Geometry check sheet. Reference: the model listing, model coordinates, mm. A direction names the side the tool comes from. Round coordinates to 2 decimals unless told otherwise and drop trailing zeros. Write each loop counter-clockwise with the first axis right and the second up, starting at its lowest first coordinate (ties: lowest second). Pieces come first, ordered by that corner, then holes. Notation, with made-up numbers: (62, 35) - (68, 35) arc R16 ccw to (68, 57) - close; hole circle Ø9 at (55.5, 37). An arc over 180 degrees is marked (long way). One line per question, with ' | ' between items. Start each with the question number.
from build123d import *

# Parameters (mm, degrees)
SKETCH_W     = 23
SKETCH_H     = 15
PAD_DEPTH    = 20
SKETCH001_R  = 2.5
PAD001_DEPTH = 1
SKETCH002_W  = 6
SKETCH002_H  = 25
PAD002_DEPTH = 20


with BuildPart() as part:
    # Sketch → Pad (new body)
    with BuildSketch(Plane.XY):
        with Locations((11.5, 0)):
            Rectangle(SKETCH_W, SKETCH_H)
    extrude(amount=PAD_DEPTH)

    # Sketch001 (on Face5 of Pad) → Pad001 (join)
    with BuildSketch(Plane(origin=(0, 0, 7), x_dir=(1, 0, 0), z_dir=(0, 0, -1))):
        with BuildLine():
            ThreePointArc((8, -13), (12.5, -17.5), (17, -13))
            Line((17, 13), (17, -13))
            ThreePointArc((17, 13), (12.5, 17.5), (8, 13))
            Line((8, -13), (8, 13))
        make_face()
        with Locations((12.5, -13)):
            Circle(SKETCH001_R, mode=Mode.SUBTRACT)
        with Locations((12.5, 13)):
            Circle(SKETCH001_R, mode=Mode.SUBTRACT)
    extrude(amount=-PAD001_DEPTH)

    # Sketch002 (on Face3 of Pad001) → Pad002 (join)
    with BuildSketch(Plane(origin=(0, 0, 0), x_dir=(1, 0, 0), z_dir=(0, 0, -1))):
        with Locations((20, 0)):
            Rectangle(SKETCH002_W, SKETCH002_H)
    extrude(amount=-PAD002_DEPTH)


solid = part.part
Q1. Go/stop test with flat-tipped pins: P1, Ø1.8, axis at x = 20.5, z = 5, coming from the -Y side; P2, Ø6.5, axis at x = 12.5, y = 13, coming from the +Z side; P3, Ø1.8, axis at x = 19.5, z = 13, coming from the +Y side. Record where each tip stops, or that it passes through.
Q2. Set-up check for faces 4 (the flat face through (8, 10.3, 7.5)), 5 (the flat face through (17, 10, 3)), 6 (the flat face through (17, -10, 3)): record each of +Z, -Z, +X, -X, +Y, -Y from which the full face is reachable in a straight line by a thin tool's end or side.
Q3. Section check B-B, the plane y = -9. Record the cut outline in (x, z).
Q4. Section check A-A, the plane z = 17. Record the cut outline in (x, y).
Q5. Thickness scan on line 1 (Y direction, x = 12.5, z = 7.5); line 2 (X direction, y = 13, z = 7.6); line 3 (Y direction, x = 10.5, z = 16.25). Record the ranges inside material, lowest first.
Q6. Section check C-C, the plane x = 17.5. Record the cut outline in (y, z), then the cut area to 3 significant figures.
Q7. Section check D-D, the plane x = 8.5. Record the cut outline in (y, z), then the cut area to 3 significant figures.
Q8. Draft check along Y on faces 1 (the cylindrical face through (10.5, 14.5, 7.5)), 2 (the flat face through (0, 0, 10)), 3 (the cylindrical face through (12.4, 17.5, 7.5)). Enter one of: pulls with the +Y half, pulls with the -Y half, needs draft (parallel to the pull), parting line crosses it, or undercut.
Result sheet:
1) P1: y = -12.5 | P2: z = 8 | P3: y = 12.5
2) face 4: +Z, -Z, -X, +Y | face 5: -Z, -X, +Y | face 6: -Z, -X, -Y
3) outline: (8, 7) - (17, 7) - (17, 0) - (23, 0) - (23, 20) - (17, 20) - (17, 8) - (8, 8) - close
4) outline: (0, -7.5) - (17, -7.5) - (17, -12.5) - (23, -12.5) - (23, 12.5) - (17, 12.5) - (17, 7.5) - (0, 7.5) - close
5) line 1: -17.5 to -15.5, -10.5 to 10.5, 15.5 to 17.5 | line 2: 8 to 10, 15 to 17 | line 3: -7.5 to 7.5
6) outline: (-12.5, 0) - (12.5, 0) - (12.5, 20) - (-12.5, 20) - close | area: 500 mm²
7) outline: (-15.06, 7) - (-7.5, 7) - (-7.5, 0) - (7.5, 0) - (7.5, 7) - (15.06, 7) - (15.06, 8) - (7.5, 8) - (7.5, 20) - (-7.5, 20) - (-7.5, 8) - (-15.06, 8) - close | area: 315 mm²
8) face 1: undercut | face 2: needs draft | face 3: pulls with the +Y half
